The figure shows three views and two pictorial views of one solid part (mm, origin at its lowest corner). Answer the questions. Coordinates: 2 decimals unless noted, no trailing zeros. Write each loop counter-clockwise with the first axis right and the second up, starting at its lowest first coordinate (ties: lowest second). Pieces come first, ordered by that corner, then holes. Notation, with made-up numbers: M 58.25,-2 L 106.25,-2 A15 cw 106.25,18 Z; hole C 4.5,32 d3. An arc over 180 degrees is marked long. Use CSV: the item, a comma, the result in double quotes.
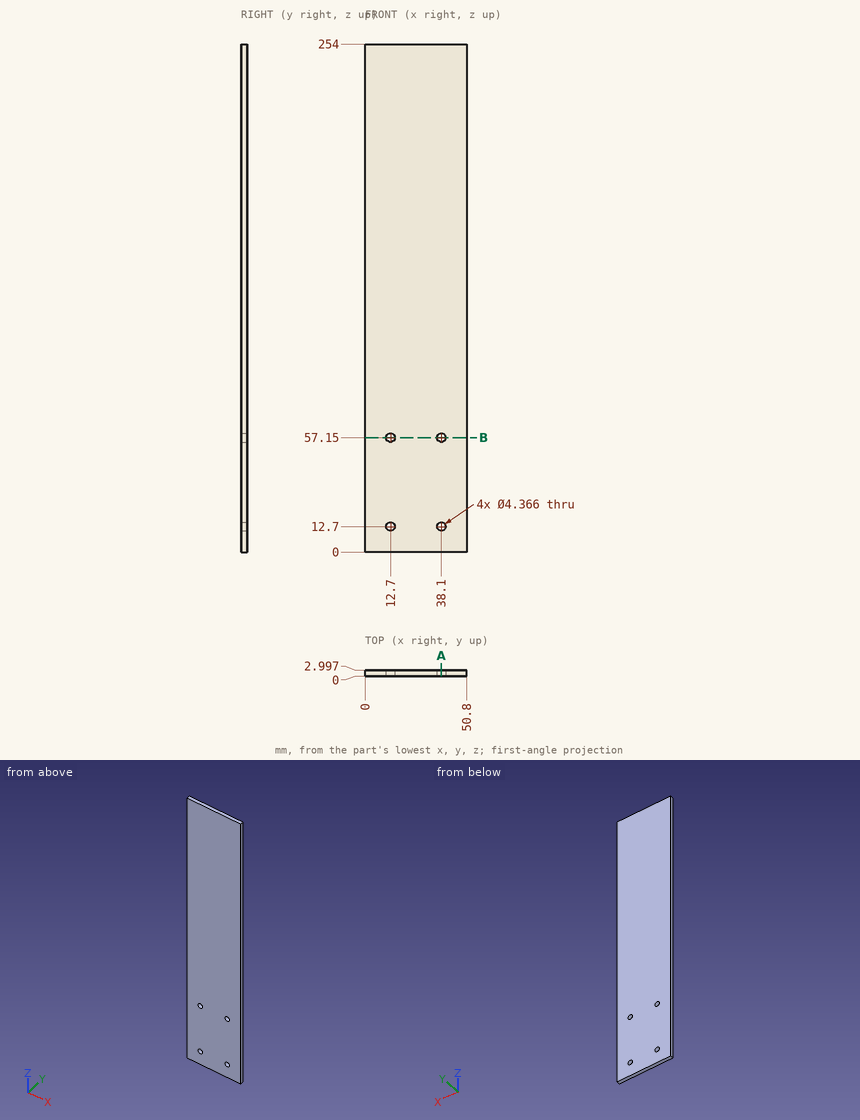
Item 1: The part is cut by section A-A (x = 38.1). Write down the section's boundary in (y, z).
Answer:
outline,"M 0,0 L 3,0 L 3,10.52 L 0,10.52 Z; M 0,14.88 L 3,14.88 L 3,54.97 L 0,54.97 Z; M 0,59.33 L 3,59.33 L 3,254 L 0,254 Z"
Item 2: The part is cut by section B-B (z = 57.15). Write down the section's boundary in (x, y).
Answer:
outline,"M 0,0 L 10.52,0 L 10.52,3 L 0,3 Z; M 14.88,0 L 35.92,0 L 35.92,3 L 14.88,3 Z; M 40.28,0 L 50.8,0 L 50.8,3 L 40.28,3 Z"
Item 3: Given pin 1 (8 mm diameter, centred on x = 25.5, z = 161, fed in from -Y); pin 2 (4 mm diameter, centred on x = 12.7, z = 57.15, fed in from +Y) (1 decimal), each flat-ended and moving along its own axis, determine where each tip first touches the part or whether it passes through.
Answer:
pin 1,"stops at y = 0"
pin 2,"passes through"
Item 4: Consider probe 1 along Z at (x, y) = (38.1, 1.65); probe 2 along Z at (x, y) = (13.5, 1.75). Determine where each line is inside the solid, lowest interval first.
Answer:
probe 1,"z = 0 to 10.52, 14.88 to 54.97, 59.33 to 254"
probe 2,"z = 0 to 10.67, 14.73 to 55.12, 59.18 to 254"
